Read the model definition and answer for the solid it produces. Units are mm, in the model's axes. Face numbers are marked on the shaded views. A direction names the side the tool comes from. Coordinates: 2 decimals unless noted, no trailing zeros. Order: outer loops, then holes, each group sorted by start corner. A loop starts at its lowest first (then second) coordinate and runs counter-clockwise, first axis right, second up.
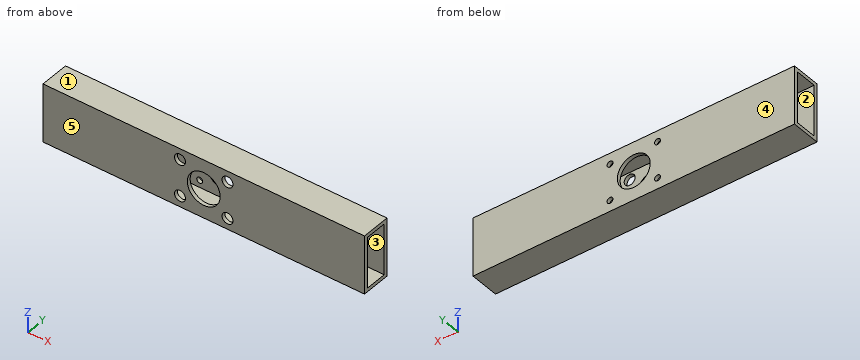
```python
from build123d import *

# Parameters (mm, degrees)
F0_W          = 25.4
F0_H          = 50.8
F0_W_2        = 19.05
F0_H_2        = 44.45
F1_DEPTH      = 139.7
F1_DEPTH_BACK = 139.7
F2_R          = 14.2875
F3_DEPTH      = 25.4
F4_R          = 2.5527
F5_DEPTH      = 25.4
F6_R          = 4.7625
F7_DEPTH      = 3.175


with BuildPart() as f1:
    # F0 (on Right) → F1 (new body, two sides)
    with BuildSketch(Plane.YZ) as f1_sk:
        with Locations((-12.7, 0)):
            Rectangle(F0_W, F0_H)
        with Locations((-12.7, 0)):
            Rectangle(F0_W_2, F0_H_2, mode=Mode.SUBTRACT)
    extrude(amount=F1_DEPTH)
    extrude(f1_sk.sketch, amount=-F1_DEPTH_BACK)

    # F2 (on Front) → F3 (cut)
    with BuildSketch(Plane.XZ):
        Circle(F2_R)
    extrude(amount=F3_DEPTH, mode=Mode.SUBTRACT)

    # F4 (on face) → F5 (cut)
    with BuildSketch(Plane.XZ.offset(25.4)):
        with Locations((20.6375, -15.875)):
            Circle(F4_R)
        with Locations((20.6375, 15.875)):
            Circle(F4_R)
        with Locations((-20.6375, 15.875)):
            Circle(F4_R)
        with Locations((-20.6375, -15.875)):
            Circle(F4_R)
    extrude(amount=-F5_DEPTH, mode=Mode.SUBTRACT)

    # F6 (on face) → F7 (cut)
    with BuildSketch(Plane.XZ.offset(25.4)):
        with Locations((20.6375, 15.875)):
            Circle(F6_R)
        with Locations((20.6375, -15.875)):
            Circle(F6_R)
        with Locations((-20.6375, -15.875)):
            Circle(F6_R)
        with Locations((-20.6375, 15.875)):
            Circle(F6_R)
    extrude(amount=-F7_DEPTH, mode=Mode.SUBTRACT)


solid = f1.part
```
1) A flat-ended cylindrical pin translates along its axis: pin 1 Ø6.5 at (x, z) = (20.64, -15.88) entering from -Y (3 decimals). Find the tip coordinate at first contact, or state that the pin passes through.
A:
pin 1: stops at y = -3.175
2) Determine the mould class of the marked faces 3, 4 and 5 for opening direction Y: pulls with the +Y half, pulls with the -Y half, needs draft (parallel to the pull), parting line crosses it, or undercut.
A:
face 3: undercut
face 4: pulls with the +Y half
face 5: pulls with the -Y half
3) A cutting plane is placed at D-D, the plane x = 41. Determine the outline of the cut face in (y, z) (3 decimals).
A:
outline: (-25.4, -25.4) - (0, -25.4) - (0, 25.4) - (-25.4, 25.4) - close; hole (-22.225, -22.225) - (-3.175, -22.225) - (-3.175, 22.225) - (-22.225, 22.225) - close
4) A cutting plane is placed at B-B, the plane z = 0. Determine the outline of the cut face in (x, y) (1 decimal), and give its area (3 significant figures).
A:
outline: (-139.7, -25.4) - (-14.3, -25.4) - (-14.3, -22.2) - (-139.7, -22.2) - close; (-139.7, -3.2) - (-14.3, -3.2) - (-14.3, 0) - (-139.7, 0) - close; (14.3, -25.4) - (139.7, -25.4) - (139.7, -22.2) - (14.3, -22.2) - close; (14.3, -3.2) - (139.7, -3.2) - (139.7, 0) - (14.3, 0) - close
area: 1,590 mm2
5) A cutting plane is placed at A-A, the plane y = -12.75. Determine the outline of the cut face in (x, z) (3 decimals), and give its area (3 significant figures).
A:
outline: (-139.7, -25.4) - (139.7, -25.4) - (139.7, -22.225) - (-139.7, -22.225) - close; (-139.7, 22.225) - (139.7, 22.225) - (139.7, 25.4) - (-139.7, 25.4) - close
area: 1,770 mm2
6) A cutting plane is placed at C-C, the plane x = 0. Determine the outline of the cut face in (y, z) (1 decimal).
A:
outline: (-25.4, -25.4) - (0, -25.4) - (0, -14.3) - (-3.2, -14.3) - (-3.2, -22.2) - (-22.2, -22.2) - (-22.2, -14.3) - (-25.4, -14.3) - close; (-25.4, 14.3) - (-22.2, 14.3) - (-22.2, 22.2) - (-3.2, 22.2) - (-3.2, 14.3) - (0, 14.3) - (0, 25.4) - (-25.4, 25.4) - close
7) Straight lines are drawn through the part: line 1 (Y direction, x = 46.5, z = -16.5) (3 decimals); line 2 (Z direction, x = -66, y = -20.75) (3 decimals); line 3 (Z direction, x = 0, y = -1.3). For each, find the intervals that lie inside material, in ascending order.
A:
line 1: y = -25.4 to -22.225, -3.175 to 0
line 2: z = -25.4 to -22.225, 22.225 to 25.4
line 3: z = -25.4 to -14.29, 14.29 to 25.4
8) Which of the six approach directions +Z, -Z, +X, -X, +Y, -Y give full straight-line access (tool end or side, diameter ignored) to the marked faces 1 and 2?
A:
face 1: +Z, +X, -X, +Y, -Y
face 2: +X, -X
